Can you work these out from the model? Positions are in its coordinate system, mm. A direction names the side the tool comes from. Coordinates: 2 decimals unless noted, no trailing zeros. Order: outer loops, then holes, each group sorted by start corner. A loop starts at its lowest first (then second) coordinate and runs counter-clockwise, first axis right, second up. Notation, with made-up numbers: (-6.75, -10.75) -> (24.25, -10.75) arc R26 cw to (24.25, 3.25) -> close; hole circle Ø4 at (59.25, 13.25). An arc over 180 degrees is marked (long way). Answer in a Markdown table with one row per item. Add a question column.
1. Imagine slicing it at B-B on z = 0.5. Write out the boundary of the cut face in (x, y).
2. If I drill on line 1 along Z through (x, y) = (2, -2.25); line 2 along Y through (x, z) = (1.5, -13); line 3 along Y through (x, z) = (1.55, -4), over which ranges is the centre line in solid material (lowest first)? Write a range as [from, to].
3. Imagine slicing it at D-D on x = 0.9. State how many separate pieces and enclosed holes the cut face has, plus the area to 3 significant figures.
4. On a 3-axis mill with a long thin cutter (end or side, diameter ignored), from which of +Z, -Z, +X, -X, +Y, -Y can I reach the whole of each face in a straight line? I mean faces 1 (the face through (1, -11, -16)), 2 (the face through (1.065, 10.715, 17.349)), 3 (the face through (1, 1.6, -13)). Say none if no direction works.
5. We'd pull the mould along Z, two halves only. Please class faces 4 (the face through (1, -2, -14.65)), 5 (the face through (1, -12.5, 14.3)), 6 (the face through (1, -12.5, -14.3)): pulls with the +Z half, pulls with the -Z half, needs draft (parallel to the pull), parting line crosses it, or undercut.
6. Imagine slicing it at A-A on y = -1.5. Write out the boundary of the cut face in (x, z), plus the area to 3 significant figures.
7. Imagine slicing it at C-C on z = 6. Write out the boundary of the cut face in (x, y), plus the area to 3 significant figures.
8. Will these pins go through, and if not, where does the flat tip stop? pin 1 (2 mm diameter, centred on y = 5.5, z = 11, fed in from -X); pin 2 (0.5 mm diameter, centred on x = 1, y = -12.5, fed in from -Z).
from build123d import *

# Parameters (mm, degrees)
SKETCH_1_W          = 18.6
SKETCH_1_H          = 11.8
SKETCH_1_R          = 1.25
EXTRUDE_1_DEPTH     = 2.1
FILLET_1_R          = 1
SKETCH_2_W          = 2
SKETCH_2_H          = 4
CUT_EXTRUDE_1_DEPTH = 10


with BuildPart() as part:
    # 草图1 → 凸台-拉伸1 (new body)
    with BuildSketch(Plane(origin=(0, 0, 0), x_dir=(0, 0, -1), z_dir=(1, 0, 0))):
        Polygon((14.3, -11), (17.65, -11), (17.65, 11), (-17.65, 11), (-17.65, -11), (-14.3, -11), (-14.3, -14), (14.3, -14), align=None)
        with BuildLine():
            ThreePointArc((-11.3, -5.55), (-11.60753788, -6.29246212), (-12.35, -6.6))
            Line((-12.35, -6.6), (-14.65, -6.6))
            ThreePointArc((-14.65, -6.6), (-15.7, -5.55), (-14.65, -4.5))
            Line((-14.65, -4.5), (-14.65, -0.5))
            ThreePointArc((-14.65, -0.5), (-15.7, 0.55), (-14.65, 1.6))
            Line((-14.65, 1.6), (-12.35, 1.6))
            ThreePointArc((-12.35, 1.6), (-11.60753788, 1.29246212), (-11.3, 0.55))
            ThreePointArc((-11.3, 0.55), (-11.60753788, -0.19246212), (-12.35, -0.5))
            Line((-12.35, -0.5), (-12.35, -4.5))
            ThreePointArc((-12.35, -4.5), (-11.60753788, -4.80753788), (-11.3, -5.55))
        make_face(mode=Mode.SUBTRACT)
        with Locations((0, -4.1)):
            Rectangle(SKETCH_1_W, SKETCH_1_H, mode=Mode.SUBTRACT)
        with BuildLine():
            ThreePointArc((15.7, -5.55), (15.39246212, -6.29246212), (14.65, -6.6))
            Line((14.65, -6.6), (12.35, -6.6))
            ThreePointArc((12.35, -6.6), (11.3, -5.55), (12.35, -4.5))
            Line((12.35, -4.5), (12.35, -0.5))
            ThreePointArc((12.35, -0.5), (11.3, 0.55), (12.35, 1.6))
            Line((12.35, 1.6), (14.65, 1.6))
            ThreePointArc((14.65, 1.6), (15.39246212, 1.29246212), (15.7, 0.55))
            ThreePointArc((15.7, 0.55), (15.39246212, -0.19246212), (14.65, -0.5))
            Line((14.65, -0.5), (14.65, -4.5))
            ThreePointArc((14.65, -4.5), (15.39246212, -4.80753788), (15.7, -5.55))
        make_face(mode=Mode.SUBTRACT)
        with Locations((-11, 5.5)):
            Circle(SKETCH_1_R, mode=Mode.SUBTRACT)
        with BuildLine():
            Line((3, 5.9), (-3, 5.9))
            ThreePointArc((-3, 5.9), (-4.05, 4.85), (-5.1, 5.9))
            Line((-5.1, 5.9), (-5.1, 8.2))
            ThreePointArc((-5.1, 8.2), (-4.05, 9.25), (-3, 8.2))
            Line((-3, 8.2), (3, 8.2))
            ThreePointArc((3, 8.2), (4.05, 9.25), (5.1, 8.2))
            Line((5.1, 8.2), (5.1, 5.9))
            ThreePointArc((5.1, 5.9), (4.05, 4.85), (3, 5.9))
        make_face(mode=Mode.SUBTRACT)
        with Locations((11, 5.5)):
            Circle(SKETCH_1_R, mode=Mode.SUBTRACT)
    extrude(amount=EXTRUDE_1_DEPTH)

    # 圆角1
    fillet_1_edges = [part.edges().sort_by_distance(p)[0] for p in [
        (1.05, -11, 17.65),
        (1.05, 11, 17.65),
        (1.05, 11, -17.65),
        (1.05, -11, -17.65),
        (1.05, -11, -14.3),
        (1.05, -14, -14.3),
        (1.05, -14, 14.3),
        (1.05, -11, 14.3),
        (1.05, -10, -9.3),
        (1.05, 1.8, -9.3),
        (1.05, 1.8, 9.3),
        (1.05, -10, 9.3),
    ]]
    fillet(fillet_1_edges, radius=FILLET_1_R)

    # 草图2 → 切除-拉伸1 (cut)
    with BuildSketch(Plane(origin=(2.1, 0, 0), x_dir=(0, 0, -1), z_dir=(1, 0, 0))):
        with Locations((0, -12)):
            Rectangle(SKETCH_2_W, SKETCH_2_H)
    extrude(amount=-CUT_EXTRUDE_1_DEPTH, mode=Mode.SUBTRACT)


solid = part.part
Answers follow:
| question | item | result |
|---|---|---|
| 1 | outline | (0, 1.8) -> (2.1, 1.8) -> (2.1, 5.9) -> (0, 5.9) -> close; (0, 8.2) -> (2.1, 8.2) -> (2.1, 11) -> (0, 11) -> close |
| 2 | line 1 | z = [-17.65, -14.65], [-12.35, -9.3], [9.3, 12.35], [14.65, 17.65] |
| 2 | line 2 | y = [-14, -6.6], [1.6, 11] |
| 2 | line 3 | y = [-14, -10], [1.8, 4.85], [9.25, 11] |
| 3 | separate pieces | 1 |
| 3 | enclosed holes | 5 |
| 3 | area | 543 mm² |
| 4 | face 1 | -Z, +X, -X, -Y |
| 4 | face 2 | +Z, +X, -X, +Y |
| 4 | face 3 | +X, -X |
| 5 | face 4 | undercut |
| 5 | face 5 | pulls with the +Z half |
| 5 | face 6 | pulls with the -Z half |
| 6 | outline | (0, -17.65) -> (2.1, -17.65) -> (2.1, -14.65) -> (0, -14.65) -> close; (0, -12.35) -> (2.1, -12.35) -> (2.1, -9.3) -> (0, -9.3) -> close; (0, 9.3) -> (2.1, 9.3) -> (2.1, 12.35) -> (0, 12.35) -> close; (0, 14.65) -> (2.1, 14.65) -> (2.1, 17.65) -> (0, 17.65) -> close |
| 6 | area | 25.4 mm² |
| 7 | outline | (0, -14) -> (2.1, -14) -> (2.1, -10) -> (0, -10) -> close; (0, 1.8) -> (2.1, 1.8) -> (2.1, 11) -> (0, 11) -> close |
| 7 | area | 27.7 mm² |
| 8 | pin 1 | passes through |
| 8 | pin 2 | stops at z = -14.3 |
